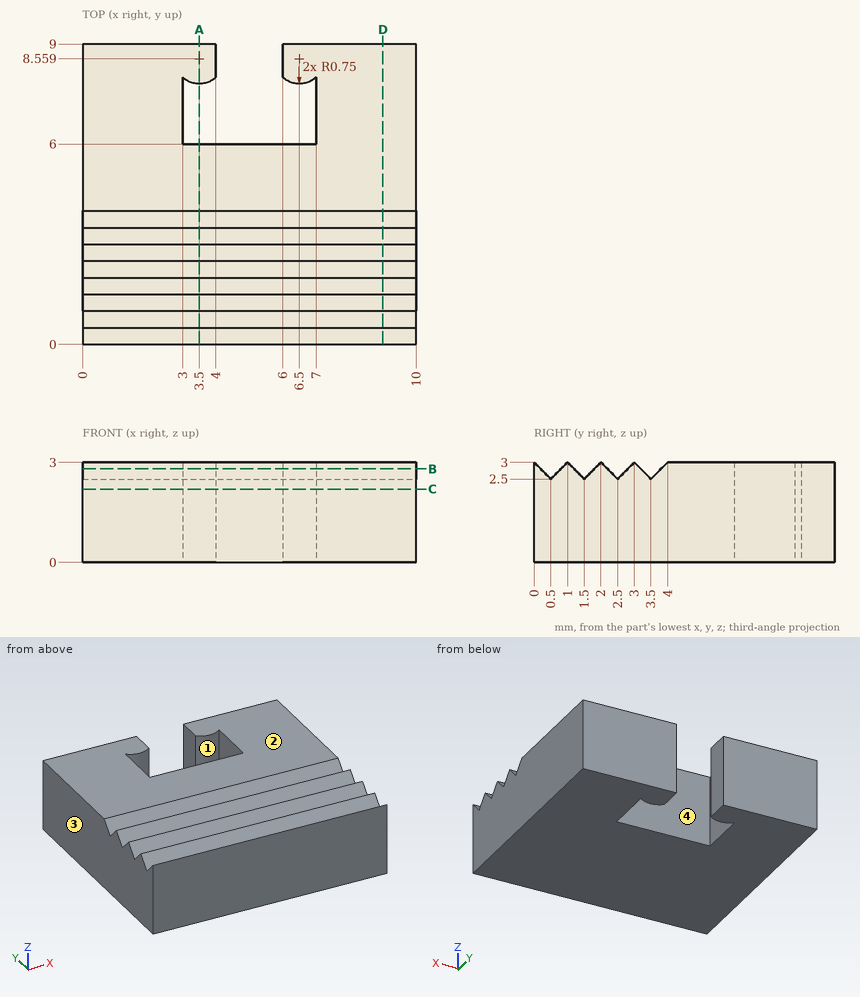
Geometry check sheet. Reference: drawing and pictorial views, mm from the part's lowest x, y, z. Round coordinates to 2 decimals unless told otherwise and drop trailing zeros. Write each loop counter-clockwise with the first axis right and the second up, starting at its lowest first coordinate (ties: lowest second). Pieces come first, ordered by that corner, then holes.
(1) Section check A-A (x = 3.5). Enter the section's corners in (y, z), plus the area to 3 significant figures.
Returned:
outline: (0, 0) - (6, 0) - (6, 3) - (4, 3) - (3.5, 2.5) - (3, 3) - (2.5, 2.5) - (2, 3) - (1.5, 2.5) - (1, 3) - (0.5, 2.5) - (0, 3) - close; (7.81, 0) - (9, 0) - (9, 3) - (7.81, 3) - close
area: 20.6 mm2
(2) Section check C-C (z = 2.2). Enter the section's corners in (x, y).
Returned:
outline: (0, 0) - (10, 0) - (10, 9) - (6, 9) - (6, 8) arc R0.75 ccw to (7, 8) - (7, 6) - (3, 6) - (3, 8) arc R0.75 ccw to (4, 8) - (4, 9) - (0, 9) - close
(3) Material ranges on line 1 (Y direction, x = 6.5, z = 0.3); line 2 (X direction, y = 7.25, z = 2.75); line 3 (Y direction, x = 2, z = 2.75), recorded low to high.
Returned:
line 1: y = 0 to 6, 7.81 to 9
line 2: x = 0 to 3, 7 to 10
line 3: y = 0 to 0.25, 0.75 to 1.25, 1.75 to 2.25, 2.75 to 3.25, 3.75 to 9
(4) Mould release check, pull along X, two halves, no side actions. Record for the marked faces 1, 2, 3 and 4: pulls with the +X half, pulls with the -X half, needs draft (parallel to the pull), parting line crosses it, or undercut.
Returned:
face 1: undercut
face 2: needs draft
face 3: pulls with the -X half
face 4: undercut
(5) Section check D-D (x = 9). Enter the section's corners in (y, z), plus the area to 3 significant figures.
Returned:
outline: (0, 0) - (9, 0) - (9, 3) - (4, 3) - (3.5, 2.5) - (3, 3) - (2.5, 2.5) - (2, 3) - (1.5, 2.5) - (1, 3) - (0.5, 2.5) - (0, 3) - close
area: 26.0 mm2
(6) Section check B-B (z = 2.8). Enter the section's corners in (x, y).
Returned:
outline: (0, 0) - (10, 0) - (10, 0.2) - (0, 0.2) - close; (0, 0.8) - (10, 0.8) - (10, 1.2) - (0, 1.2) - close; (0, 1.8) - (10, 1.8) - (10, 2.2) - (0, 2.2) - close; (0, 2.8) - (10, 2.8) - (10, 3.2) - (0, 3.2) - close; (0, 3.8) - (10, 3.8) - (10, 9) - (6, 9) - (6, 8) arc R0.75 ccw to (7, 8) - (7, 6) - (3, 6) - (3, 8) arc R0.75 ccw to (4, 8) - (4, 9) - (0, 9) - close
